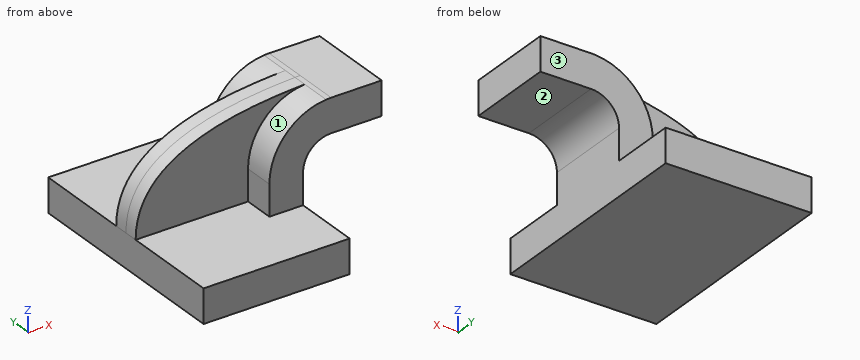
from build123d import *

# Parameters (mm, degrees)
F1_DEPTH = 63.5
F0_W     = 25.4
F0_H     = 19.05
F2_DEPTH = 25.4
F3_DEPTH = 7.9375


with BuildPart() as f1:
    # F0 (on Front) → F1 (new body, symmetric)
    with BuildSketch(Plane.XZ):
        Polygon((-30.89006, -22.216722), (-94.39006, -22.216722), (-94.39006, -41.266722), (-11.84006, -41.266722), (-11.84006, -22.216722), align=None)
    extrude(amount=F1_DEPTH, both=True)

    # F0 (on Front) → F2 (join, symmetric)
    with BuildSketch(Plane.XZ):
        with BuildLine():
            Line((-30.89006, -4.741522), (-30.89006, -22.216722))
            Line((-30.89006, -22.216722), (-11.84006, -22.216722))
            Line((-11.84006, -22.216722), (-11.84006, -4.741522))
            ThreePointArc((-11.84006, -4.741522), (-7.19038, 6.483798), (4.03494, 11.133478))
            Line((4.03494, 11.133478), (7.20994, 11.133478))
            Line((7.20994, 11.133478), (7.20994, 30.183478))
            Line((7.20994, 30.183478), (4.03494, 30.183478))
            add(Edge.make_bspline(
                [(1.159366, 30.064896), (2.145677, 30.107801), (3.105038, 30.147007), (4.03494, 30.183478)],
                knots=[108.256828, 108.256828, 108.256828, 108.256828, 111.504536, 111.504536, 111.504536, 111.504536], degree=3))
            ThreePointArc((1.159366, 30.064896), (-21.657326, 18.915678), (-30.89006, -4.741522))
        make_face()
        with Locations((19.90994, 20.658478)):
            Rectangle(F0_W, F0_H)
    extrude(amount=F2_DEPTH, both=True)

    # F0 (on Front) → F3 (join, symmetric)
    with BuildSketch(Plane.XZ):
        with BuildLine():
            add(Edge.make_bspline(
                [(-94.39006, -22.216722), (-94.538549, 23.095014), (-31.717619, 28.634726), (1.159366, 30.064896)],
                knots=[0, 0, 0, 0, 108.256828, 108.256828, 108.256828, 108.256828], degree=3))
            Line((-94.39006, -22.216722), (-30.89006, -22.216722))
            Line((-30.89006, -22.216722), (-30.89006, -4.741522))
            ThreePointArc((-30.89006, -4.741522), (-21.657326, 18.915678), (1.159366, 30.064896))
        make_face()
    extrude(amount=F3_DEPTH, both=True)


solid = f1.part
The model under review builds one solid part; all positions refer to its coordinate system, in mm. Face numbers are marked on the shaded views. A direction names the side the tool comes from. Give positions to 0.01 mm unless a question says otherwise; leave off trailing zeros. Order: outer loops, then holes, each group sorted by start corner. A loop starts at its lowest first (then second) coordinate and runs counter-clockwise, first axis right, second up. Notation, with made-up numbers: M 46.25,-36.75 L 51.25,-36.75 A19 ccw 51.25,-20.75 Z; hole C 73,-2 d3. An arc over 180 degrees is marked long. Use one line per item in the form item = value. Start each with the question number.
Item 1: We need section A-A on x = 8. Give the boundary of the cut face in (y, z).
Item 2: For the marked faces 1, 2 and 3, list the 3-axis set-ups (+Z, -Z, +X, -X, +Y, -Y) from which the entire face can be reached by the end or side of a thin tool; tool diameter is ignored.
Item 3: We need section B-B on y = 29. Give the boundary of the cut face in (x, z), plus the area to 3 significant figures.
Item 4: Insertion check: pin 1 Ø6 at (x, y) = (-17, -28.5) entering from +Z; pin 2 Ø14.5 at (x, y) = (20, -10) entering from -Z; pin 3 Ø6 at (x, z) = (-30, -2.5) entering from +Y. Each pin has a flat end and moves straight along its axis. Give the tip position at first contact, or say it passes through.
Item 5: To check wall thickness, follow line 1 along X through (y, z) = (-56, -25); line 2 along Y through (x, z) = (1, 25.5); line 3 along X through (y, z) = (19.5, -12). State the ranges of each line that lie inside material, in increasing order. Write a range as from..to.
Completed:
q1.outline = M -25.4,11.13 L 25.4,11.13 L 25.4,30.18 L -25.4,30.18 Z
q2.face_1 = +Z, -X, -Y
q2.face_2 = -Z, +X, +Y, -Y
q2.face_3 = +Z, +X, -X, +Y
q3.outline = M -94.39,-41.27 L -11.84,-41.27 L -11.84,-22.22 L -94.39,-22.22 Z
q3.area = 1,570 mm²
q4.pin_1 = -22.22
q4.pin_2 = 11.13
q4.pin_3 = 25.4
q5.line_1 = -94.39..-11.84
q5.line_2 = -25.4..25.4
q5.line_3 = -30.89..-11.84
